Autodesk Inventor part; units mm, degrees
ref_plane "YZ Plane" through (0, 0, 0) normal (1, 0, 0) x (0, 1, 0)
ref_plane "XZ Plane" through (0, 0, 0) normal (0, 1, 0) x (-1, 0, 0)
ref_plane "XY Plane" through (0, 0, 0) normal (0, 0, 1) x (1, 0, 0)
sketch "Sketch1" plane through (0, 0, 0) normal (0, 1, 0) x (-1, 0, 0)
  point P0 (0, 0)
sketch "Sketch2" plane through (0, 0, 0) normal (0, 0, 1) x (1, 0, 0)
  line L0 (0, 0) -> (150, 0)
  line L1 (150, 0) -> (150, -100)
  line L2 (150, -100) -> (0, -100)
  line L3 (0, -100) -> (0, 0)
extrude "Extrusion1" add sketch "Sketch2" along normal blind 150
sketch "Sketch3" plane through (150, -100, 0) normal (1, 0, 0) x (0, 0, -1)
  circle A0 centre (-74.7614, 78.8048) radius 15
  point P0 (0, 100)
  dimension "d4" = 30
extrude "Extrusion2" cut sketch "Sketch3" against normal blind 40.75
sketch "Sketch4" plane through (0, 0, 0) normal (0, 1, 0) x (1, 0, 0)
  line L0 (57.0345, -48.171) -> (77.0345, -48.171)
  line L1 (77.0345, -48.171) -> (77.0345, -112.9129)
  line L2 (77.0345, -112.9129) -> (57.0345, -112.9129)
  line L3 (57.0345, -112.9129) -> (57.0345, -48.171)
  point P0 (0, 0)
extrude "Extrusion3" add sketch "Sketch4" along normal blind 22
properties part number "water tank 1" material "PVC, Unplasticized"
Build history of the part. All positions in model axes, mm. A direction names the side the tool comes from. Round coordinates to 2 decimals unless told otherwise and drop trailing zeros. Write each loop counter-clockwise with the first axis right and the second up, starting at its lowest first coordinate (ties: lowest second). Pieces come first, ordered by that corner, then holes.
1) Drill centre lines: probe 1 along Y at (x, z) = (82, 21); probe 2 along Y at (x, z) = (144.5, 73). Where is each one in solid material? Low to high.
2) Mould opens along Z. For faces 1 (the flat face through (109.25, -21, 75)), 2 (the cylindrical face through (129.91, -26.94, 60.905)), 3 (the flat face through (67, 11, 48.171)), 4 (the flat face through (77.034, 11, 80)) say: +Z half, -Z half, draft (parallel to the pull), parting line (faces both ways), or undercut.
3) Pin check, flat tips, straight feed: pin 1 (24 mm diameter, centred on y = -22, z = 76, fed in from +X); pin 2 (6 mm diameter, centred on x = 71.5, y = 8.5, fed in from -Z); pin 3 (12 mm diameter, centred on x = 109.5, z = 38, fed in from +Y). Stop position of each tip, or through.
4) Band-saw the part on A-A, the plane x = 67. List the corners of the cut face in (y, z), and give its area (3 significant figures).
5) Band-saw the part on B-B, the plane z = 64. List the corners of the cut face in (x, y), and give its area (3 significant figures).
6) Band-saw the part on C-C, the plane y = -8.5. List the corners of the cut face in (x, z).
7) 3-axis set-ups, long thin cutter, end or side, ignore diameter. For faces 5 (the flat face through (76, -100, 74)), 6 (the flat face through (57.034, 11, 81)), 7 (the flat face through (67, 11, 112.913)): which of +Z, -Z, +X, -X, +Y, -Y reach the whole face in a straight line?
8) Band-saw the part on D-D, the plane x = 116. List the corners of the cut face in (y, z), and give its area (3 significant figures).
Ans:
1. probe 1: y = -100 to 0
1. probe 2: y = -100 to -36.09, -6.3 to 0
2. face 1: undercut
2. face 2: undercut
2. face 3: -Z half
2. face 4: draft
3. pin 1: stops at x = 109.25
3. pin 2: stops at z = 48.17
3. pin 3: stops at y = 0
4. outline: (-100, 0) - (0, 0) - (0, 48.17) - (22, 48.17) - (22, 112.91) - (0, 112.91) - (0, 150) - (-100, 150) - close
4. area: 16,400 mm2
5. outline: (0, -100) - (150, -100) - (150, -31.64) - (109.25, -31.64) - (109.25, -10.75) - (150, -10.75) - (150, 0) - (77.03, 0) - (77.03, 22) - (57.03, 22) - (57.03, 0) - (0, 0) - close
5. area: 14,600 mm2
6. outline: (0, 0) - (150, 0) - (150, 66.77) - (109.25, 66.77) - (109.25, 82.75) - (150, 82.75) - (150, 150) - (0, 150) - close
7. face 5: +Z, -Z, +X, -X, -Y
7. face 6: +Z, -Z, -X, +Y
7. face 7: +Z, +X, -X, +Y
8. outline: (-100, 0) - (0, 0) - (0, 150) - (-100, 150) - close; hole circle Ø30 at (-21.2, 74.76)
8. area: 14,300 mm2
